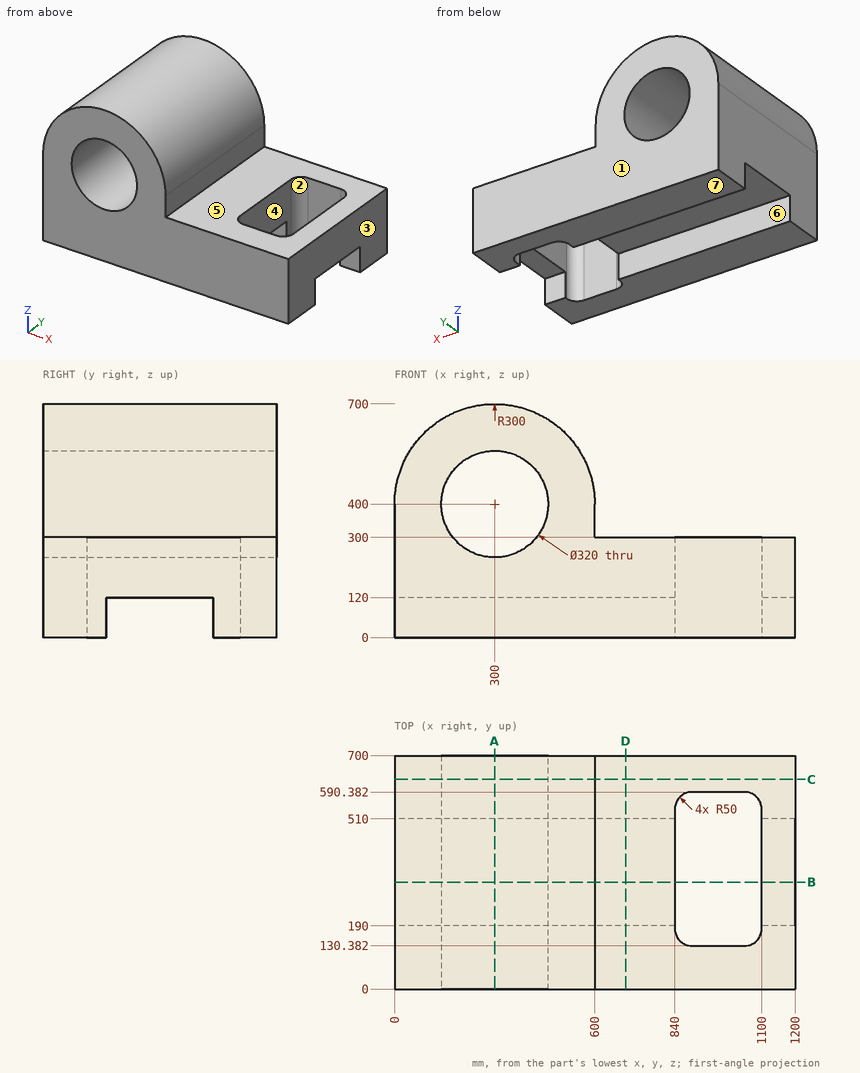
Print and shaded views of the part. All mm, measured from the part's lowest x, y and z. A direction names the side the tool comes from. Coordinates: 2 decimals unless noted, no trailing zeros. Loops run counter-clockwise (first coordinate to the right, second up) from the corner with the lowest first, then second, coordinate; pieces in that order, holes last. Notation, with made-up numbers: (81.25, 38) - (129.25, 38) arc R33 cw to (129.25, 77) - close; hole circle Ø2 at (62.25, 53.25). An arc over 180 degrees is marked (long way). Use one line per item in the form item = value. Start each with the question number.
1) Drill centre lines: L1, parallel to Z at x = 300, y = 426; L2, parallel to Y at x = 530.5, z = 102.5; L3, parallel to X at y = 492.5, z = 238. Where is each one in solid material? Low to high. Write a range as from..to.
2) Band-saw the part on A-A (x = 300). Give the cut face in (y, z).
3) Band-saw the part on D-D (x = 692.5). Give the cut face in (y, z), and give its area (3 significant figures).
4) Band-saw the part on C-C (y = 629). Give the cut face in (x, z).
5) Two-plate mould, pull along Y, no slides. Class the marked faces 1, 2 and 3: +Y half, -Y half, draft (parallel to the pull), parting line (faces both ways), or undercut.
6) Tool access for the marked faces 4, 5, 6 and 7: list every direction of +Z, -Z, +X, -X, +Y, -Y with a clear straight run to the whole face (end or side of a thin tool).
7) Flat gauge pins, fed straight in: pin 1 (1.5 mm diameter, centred on x = 788, y = 495.5, fed in from +Z); pin 2 (12 mm diameter, centred on x = 322, y = 326, fed in from +Z); pin 3 (6 mm diameter, centred on y = 399.5, z = 585, fed in from +X). Where does each tip first touch, or does it go through?
8) Band-saw the part on B-B (y = 321). Give the cut face in (x, z).
Check values:
q1.L1 = 120..240, 560..700
q1.L2 = 0..190, 510..700
q1.L3 = 0..840, 1100..1200
q2.outline = (0, 0) - (190, 0) - (190, 120) - (510, 120) - (510, 0) - (700, 0) - (700, 240) - (0, 240) - close; (0, 560) - (700, 560) - (700, 700) - (0, 700) - close
q3.outline = (0, 0) - (190, 0) - (190, 120) - (510, 120) - (510, 0) - (700, 0) - (700, 300) - (0, 300) - close
q3.area = 172,000 mm2
q4.outline = (0, 0) - (1200, 0) - (1200, 300) - (600, 300) - (600, 400) arc R300 ccw to (0, 400) - close; hole circle Ø320 at (300, 400)
q5.face_1 = +Y half
q5.face_2 = undercut
q5.face_3 = draft
q6.face_4 = +Z, -Z
q6.face_5 = +Z, +X, +Y, -Y
q6.face_6 = -Z, +X, -X
q6.face_7 = -Z, +X, -X, +Y, -Y
q7.pin_1 = 300
q7.pin_2 = 699.57
q7.pin_3 = 538.49
q8.outline = (0, 120) - (840, 120) - (840, 300) - (600, 300) - (600, 400) arc R300 ccw to (0, 400) - close; (1100, 120) - (1200, 120) - (1200, 300) - (1100, 300) - close; hole circle Ø320 at (300, 400)
